Drawing for the job (mm, zero at the part's lowest x, y, z). Round coordinates to 2 decimals unless told otherwise and drop trailing zeros. Write each loop counter-clockwise with the first axis right and the second up, starting at its lowest first coordinate (ties: lowest second). Pieces come first, ordered by that corner, then holes. Notation, with made-up numbers: (36.25, 8) -> (56.25, 8) arc R19 ccw to (56.25, 43) -> close; hole circle Ø9 at (-30, -22). An arc over 180 degrees is marked (long way). Answer in a Markdown table with one row per item. Add a question column.
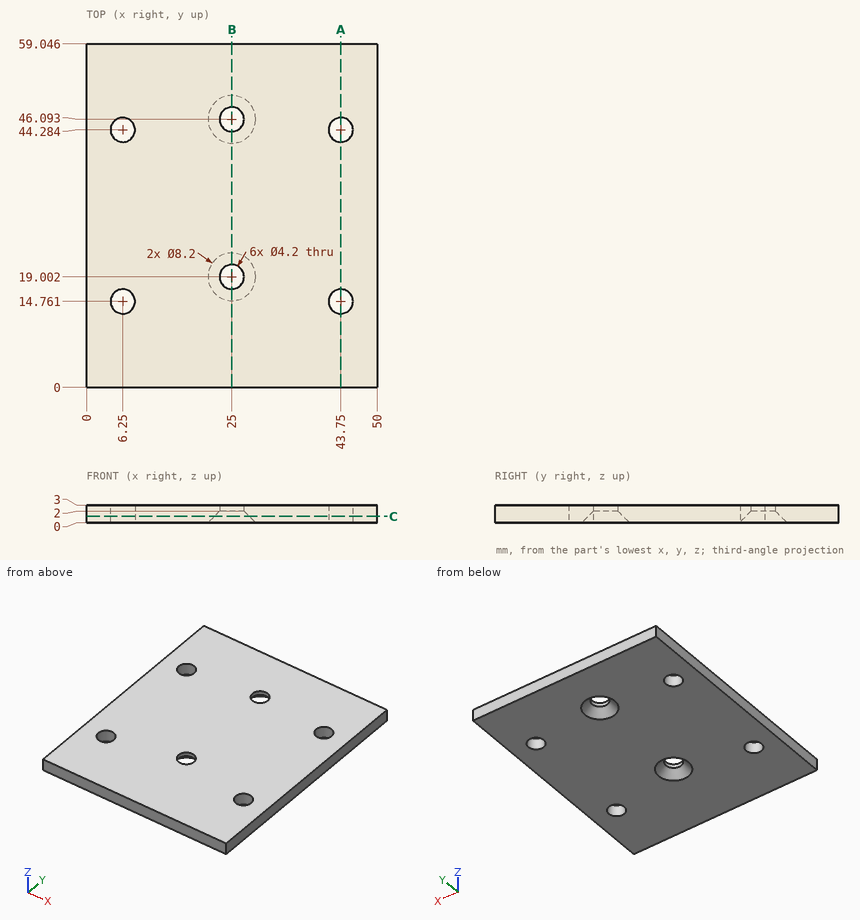
(1) Probe line 1 along Y through (x, z) = (43.75, 0.85) (1 decimal); line 2 along Y through (x, z) = (25, 2.6) (1 decimal); line 3 along X through (y, z) = (19, 2.3). List the from-to ranges inside material, lowest first.
(2) Saw through at C-C (z = 1.1). Count the separate pieces of the cut face and the enclosed holes in it, plus the area to 3 significant figures.
(3) Saw through at B-B (x = 25). List the corners of the cut face in (y, z) (1 decimal).
(4) Drop flat-ended pins along their axis: P1, Ø6.5, axis at x = 25, y = 46.09, coming from the -Z side; P2, Ø1, axis at x = 9, y = 33.5, coming from the -Z side. Give the stop position or say it passes through.
(5) Saw through at A-A (x = 43.75). List the corners of the cut face in (y, z) (1 decimal).
Answer sheet:
| question | item | result |
|---|---|---|
| 1 | line 1 | y = 0 to 12.7, 16.9 to 42.2, 46.4 to 59 |
| 1 | line 2 | y = 0 to 16.9, 21.1 to 44, 48.2 to 59 |
| 1 | line 3 | x = 0 to 22.9, 27.1 to 50 |
| 2 | separate pieces | 1 |
| 2 | enclosed holes | 6 |
| 2 | area | 2,840 mm² |
| 3 | outline | (0, 0) -> (14.9, 0) -> (16.9, 2) -> (16.9, 3) -> (0, 3) -> close; (21.1, 2) -> (23.1, 0) -> (42, 0) -> (44, 2) -> (44, 3) -> (21.1, 3) -> close; (48.2, 2) -> (50.2, 0) -> (59, 0) -> (59, 3) -> (48.2, 3) -> close |
| 4 | P1 | stops at z = 0.85 |
| 4 | P2 | stops at z = 0 |
| 5 | outline | (0, 0) -> (12.7, 0) -> (12.7, 3) -> (0, 3) -> close; (16.9, 0) -> (42.2, 0) -> (42.2, 3) -> (16.9, 3) -> close; (46.4, 0) -> (59, 0) -> (59, 3) -> (46.4, 3) -> close |
